Design review of the part built by this model. Coordinates are the model's own, in mm. Face numbers are marked on the shaded views. Give positions to 0.01 mm unless a question says otherwise; leave off trailing zeros. Loops run counter-clockwise (first coordinate to the right, second up) from the corner with the lowest first, then second, coordinate; pieces in that order, holes last. Notation, with made-up numbers: (89.5, -31.75) -> (145.5, -31.75) arc R31 cw to (145.5, -1.75) -> close; hole circle Ø6 at (18, 67.25). An arc over 180 degrees is marked (long way). Answer in a Markdown table with one row per item. Add a question column.
(1) For line 1 (Y direction, x = 3.5, z = 2.55); line 2 (Y direction, x = 0, z = 2.5); line 3 (Y direction, x = 3.1, z = 0.85), list the stretches that pass through material, from the lowest coordinate up.
(2) Consider section C-C on x = 3.1. Write out the cut boundary in (y, z).
(3) Consider section B-B on y = 0. Write out the cut boundary in (x, z), then the cut area to 3 significant figures.
(4) Consider section A-A on x = 0. Write out the cut boundary in (y, z), then the cut area to 3 significant figures.
(5) Consider section D-D on z = 1.25. Write out the cut boundary in (x, y).
(6) Draft analysis for pull direction Y (two halves, no side actions). For the marked faces 1, 2 and 3, state which applies: +Y half, -Y half, draft (parallel to the pull), parting line (faces both ways), or undercut.
Autodesk Inventor part; units mm, degrees
ref_plane "YZ Plane" through (0, 0, 0) normal (1, 0, 0) x (0, 1, 0)
ref_plane "XZ Plane" through (0, 0, 0) normal (0, 1, 0) x (-1, 0, 0)
ref_plane "XY Plane" through (0, 0, 0) normal (0, 0, 1) x (1, 0, 0)
sketch "Sketch1" plane through (0, 0, 0) normal (0, 0, 1) x (1, 0, 0)
  point P0 (0, 0)
sketch "Sketch2" plane through (0, 0, 0) normal (0, 0, 1) x (1, 0, 0)
  circle A0 centre (0, 0) radius 11
  circle A1 centre (0, 0) radius 2
  circle A2 centre (-6.2, 0) radius 1.5
  circle A3 centre (0, 0) radius 6.2 construction
  circle A4 centre (3.1, -5.3694) radius 1.5
  circle A5 centre (3.1, 5.3694) radius 1.5
  dimension "d3" = 12.4
  dimension "d0" = 22
  dimension "d1" = 4
  dimension "d2" = 3
  dimension "d6" = 360
extrude "Extrusion1" add sketch "Sketch2" along normal blind 3
properties part number "WheelAdapter-4mm-2" material "Aluminum 6061"
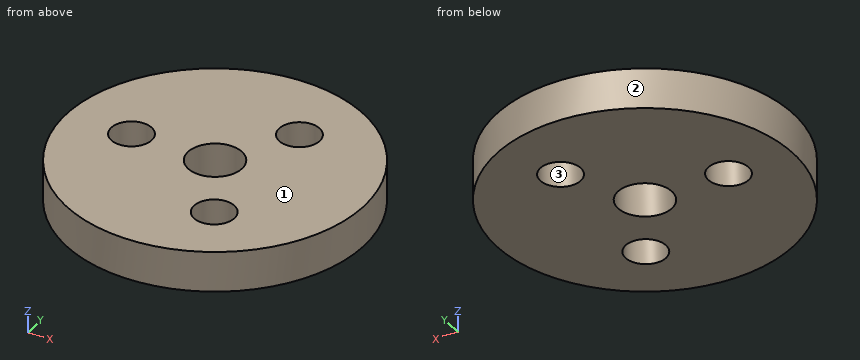
Values follow:
| question | item | result |
|---|---|---|
| 1 | line 1 | -10.43 to -6.82, -3.92 to 3.92, 6.82 to 10.43 |
| 1 | line 2 | -11 to -2, 2 to 11 |
| 1 | line 3 | -10.55 to -6.87, -3.87 to 3.87, 6.87 to 10.55 |
| 2 | outline | (-10.55, 0) -> (-6.87, 0) -> (-6.87, 3) -> (-10.55, 3) -> close; (-3.87, 0) -> (3.87, 0) -> (3.87, 3) -> (-3.87, 3) -> close; (6.87, 0) -> (10.55, 0) -> (10.55, 3) -> (6.87, 3) -> close |
| 3 | outline | (-11, 0) -> (-7.7, 0) -> (-7.7, 3) -> (-11, 3) -> close; (-4.7, 0) -> (-2, 0) -> (-2, 3) -> (-4.7, 3) -> close; (2, 0) -> (11, 0) -> (11, 3) -> (2, 3) -> close |
| 3 | area | 45.0 mm2 |
| 4 | outline | (-11, 0) -> (-2, 0) -> (-2, 3) -> (-11, 3) -> close; (2, 0) -> (11, 0) -> (11, 3) -> (2, 3) -> close |
| 4 | area | 54.0 mm2 |
| 5 | outline | circle Ø22 at (0, 0); hole circle Ø3 at (-6.2, 0); hole circle Ø4 at (0, 0); hole circle Ø3 at (3.1, -5.37); hole circle Ø3 at (3.1, 5.37) |
| 6 | face 1 | draft |
| 6 | face 2 | parting line |
| 6 | face 3 | undercut |
